Check sheet for the modelled part. Datum: model origin and axes. Units: mm. A direction names the side the tool comes from. Give positions to 0.01 mm unless a question says otherwise; leave off trailing zeros. Loops run counter-clockwise (first coordinate to the right, second up) from the corner with the lowest first, then second, coordinate; pieces in that order, holes last. Notation, with made-up numbers: M 18.5,82 L 59.5,82 A36 ccw 59.5,120 Z; hole C -5,1 d6. An arc over 180 degrees is marked long. Write each question's results on one line, items separated by ' | '. Start each with the question number.
1. Sectioned sample at B-B on x = -350. Record the cut outline in (y, z), and give its area (3 significant figures).
2. Go/stop test with a flat-tipped pin: pin 1 (1 mm diameter, centred on y = 12, z = 147, fed in from -X). Record where the tip stops, or that it passes through.
3. Sectioned sample at C-C on y = 14.5. Record the cut outline in (x, z).
4. Tool access check on faces 1 (the flat face through (-351, 20, 99)), 2 (the cylindrical face through (-312.368, 14.93, 40.976)). Record the directions out of +Z, -Z, +X, -X, +Y, -Y that give a thin tool (end or side, any length) a straight path to the whole face; none if there is none.
5. Sectioned sample at A-A on z = 100. Record the cut outline in (x, y), and give its area (3 significant figures).
6. Material ranges on line 1 along Y through (x, z) = (-195, -88); line 2 along X through (y, z) = (16.5, 119), recorded low to high.
7. Sectioned sample at D-D on x = 136. Record the cut outline in (y, z), and give its area (3 significant figures).
```python
from build123d import *

# Parameters (mm, degrees)
SKETCH1_W           = 1000
SKETCH1_H           = 500
BOSS_EXTRUDE1_DEPTH = 10
SKETCH2_R           = 70
BOSS_EXTRUDE2_DEPTH = 10


with BuildPart() as part:
    # Sketch1 → Boss-Extrude1 (new body)
    with BuildSketch(Plane(origin=(0, 0, 0), x_dir=(1, 0, 0), z_dir=(0, 1, 0))):
        Rectangle(SKETCH1_W, SKETCH1_H)
    extrude(amount=BOSS_EXTRUDE1_DEPTH)

    # Sketch2 → Boss-Extrude2 (add)
    with BuildSketch(Plane(origin=(0, 10, 0), x_dir=(1, 0, 0), z_dir=(0, 1, 0))):
        with Locations((-350, -100)):
            Circle(SKETCH2_R)
    extrude(amount=BOSS_EXTRUDE2_DEPTH)


solid = part.part
```
Output values:
1) outline: M 0,-250 L 10,-250 L 10,30 L 20,30 L 20,170 L 10,170 L 10,250 L 0,250 Z | area: 6,400 mm2
2) pin 1: x = -402.32
3) outline: C -350,100 d140
4) face 1: +Z, -Z, +X, -X, +Y | face 2: +Y
5) outline: M -500,0 L 500,0 L 500,10 L -280,10 L -280,20 L -420,20 L -420,10 L -500,10 Z | area: 11,400 mm2
6) line 1: 0 to 10 | line 2: -417.37 to -282.63
7) outline: M 0,-250 L 10,-250 L 10,250 L 0,250 Z | area: 5,000 mm2
